from build123d import *

# Parameters (mm, degrees)
BOSS_EXTRUDE1_DEPTH = 9
CUT_EXTRUDE1_DEPTH  = 7
CUT_EXTRUDE2_DEPTH  = 2.6
BOSS_EXTRUDE2_DEPTH = 3


with BuildPart() as part:
    # Sketch1 → Boss-Extrude1 (new body, symmetric)
    with BuildSketch(Plane.XY):
        Polygon((0, 0), (0, 18), (3, 18), (18, 3), (18, 0), align=None)
    extrude(amount=BOSS_EXTRUDE1_DEPTH, both=True)

    # Sketch2 → Cut-Extrude1 (cut, symmetric)
    with BuildSketch(Plane.XY):
        Polygon((3, 18), (3, 3), (18, 3), align=None)
    extrude(amount=CUT_EXTRUDE1_DEPTH, both=True, mode=Mode.SUBTRACT)

    # Sketch3 → Cut-Extrude2 (cut, symmetric)
    with BuildSketch(Plane.XY):
        Polygon((0, 14), (3, 14), (3, 7), (0, 4), align=None)
        Polygon((7, 3), (14, 3), (14, 0), (4, 0), align=None)
    extrude(amount=CUT_EXTRUDE2_DEPTH, both=True, mode=Mode.SUBTRACT)

    # Sketch4 → Boss-Extrude2 (add, symmetric)
    with BuildSketch(Plane.XY):
        Polygon((1.497483368, -1.80628538), (0.504853677, -0.797938337), (1.234750477, 0), (3.535533906, 0), align=None)
        Polygon((0, 3.535533906), (-1.80628538, 1.497483368), (-0.797938337, 0.504853677), (0, 1.234750477), align=None)
        Polygon((0, 17.3), (0, 14.999216572), (-0.797938337, 14.269319771), (-1.80628538, 15.261949462), align=None)
        Polygon((14.999216572, 0), (14.269319771, -0.797938337), (15.261949462, -1.80628538), (17.3, 0), align=None)
    extrude(amount=BOSS_EXTRUDE2_DEPTH, both=True)


solid = part.part
Verification items for the finished model (mm, model axes). A direction names the side the tool comes from. Round coordinates to 2 decimals unless told otherwise and drop trailing zeros. Order: outer loops, then holes, each group sorted by start corner. A loop starts at its lowest first (then second) coordinate and runs counter-clockwise, first axis right, second up.
1. Release check for a two-part mould opening along Z. For faces 1 (the flat face through (15, -1, 3)), 2 (the flat face through (10, 2, -2.6)), 3 (the flat face through (1, 14, 0)), 4 (the flat face through (18, 2, 0)) record: +Z half, -Z half, draft (parallel to the pull), parting line (faces both ways), or undercut.
Final values:
face 1: +Z half
face 2: undercut
face 3: undercut
face 4: draft
2. Section check D-D on y = 5.25. Record the cut outline in (x, z), then the cut area to 3 significant figures.
Final values:
outline: (0, -9) - (15.75, -9) - (15.75, -7) - (3, -7) - (3, 7) - (15.75, 7) - (15.75, 9) - (0, 9) - (0, 2.6) - (1.25, 2.6) - (1.25, -2.6) - (0, -2.6) - close
area: 98.5 mm2
3. Section check B-B on y = 12.5. Record the cut outline in (x, z).
Final values:
outline: (0, -9) - (8.5, -9) - (8.5, -7) - (3, -7) - (3, -2.6) - (0, -2.6) - close; (0, 2.6) - (3, 2.6) - (3, 7) - (8.5, 7) - (8.5, 9) - (0, 9) - close
4. Thickness scan on L1, parallel to Z at x = 7.5, y = 2.75; L2, parallel to Z at x = 3.25, y = 6; L3, parallel to X at y = 5.25, z = 4.5. Record the ranges inside material, lowest first.
Final values:
L1: z = -9 to -2.6, 2.6 to 9
L2: z = -9 to -7, 7 to 9
L3: x = 0 to 3
5. Access from +Z, -Z, +X, -X, +Y, -Y to the whole of each face (thin tool, end or side, straight path). Record for faces 5 (the flat face through (14.759, -1.295, 0.042)), 6 (the flat face through (2, 10, 2.6)), 7 (the flat face through (15, -1, -3)), 8 (the flat face through (14, 2, 0)).
Final values:
face 5: +Z, -Z, -Y
face 6: -X
face 7: -Z, +X, -X, -Y
face 8: +Y, -Y
6. Go/stop test with flat-tipped pins: P1, Ø1.5, axis at y = 5, z = 5, coming from the +X side; P2, Ø2, axis at y = 14, z = 1.5, coming from the -X side; P3, Ø6, axis at y = 15, z = 6.5, coming from the +X side. Record where each tip stops, or that it passes through.
Final values:
P1: stops at x = 3
P2: stops at x = -1.54
P3: stops at x = 8.96
7. Section check C-C on z = 1.5. State how many separate pieces and enclosed holes the cut face has, then the cut area to 3 significant figures.
Final values:
separate pieces: 3
enclosed holes: 0
area: 59.4 mm2
8. Section check A-A on x = 8.75. Record the cut outline in (y, z), then the cut area to 3 significant figures.
Final values:
outline: (0, -9) - (12.25, -9) - (12.25, -7) - (3, -7) - (3, -2.6) - (0, -2.6) - close; (0, 2.6) - (3, 2.6) - (3, 7) - (12.25, 7) - (12.25, 9) - (0, 9) - close
area: 75.4 mm2
